Input: part model. Units: mm. Frame: model coordinates. Face numbers are marked on the shaded views. Give positions to 0.01 mm unless a question says otherwise; leave off trailing zeros. Loops run counter-clockwise (first coordinate to the right, second up) from the corner with the lowest first, then second, coordinate; pieces in that order, holes last. Notation, with made-up numbers: (-20.5, -29.5) - (-5.5, -29.5) arc R18 ccw to (-5.5, -17.5) - close; hole circle Ø8 at (21.5, 30). An arc over 180 degrees is marked (long way). Answer as a JSON object with one key per item and string values.
from build123d import *

# Parameters (mm, degrees)
SKETCH1_W           = 340.2
SKETCH1_H           = 155
BOSS_EXTRUDE1_DEPTH = 2
SKETCH2_R           = 2.5
CUT_EXTRUDE1_DEPTH  = 3
LPATTERN1_COUNT     = 4
LPATTERN1_PITCH     = 10
SKETCH3_W           = 59.862571915
SKETCH3_H           = 20.5
CUT_EXTRUDE2_DEPTH  = 3
LPATTERN2_COUNT     = 5
LPATTERN2_PITCH     = 10
SKETCH4_W           = 59.862571915
SKETCH4_H           = 9.012650354
CUT_EXTRUDE3_DEPTH  = 3
FILLET1_R           = 10
FILLET2_R           = 10
CUT_EXTRUDE4_DEPTH  = 3


with BuildPart() as part:
    # Sketch1 → Boss-Extrude1 (new body)
    with BuildSketch(Plane.XY):
        with Locations((440, -1022.5)):
            Rectangle(SKETCH1_W, SKETCH1_H)
    extrude(amount=BOSS_EXTRUDE1_DEPTH)

    # Sketch2 → Cut-Extrude1 (cut, through all)
    with BuildSketch(Plane.XY.offset(2)):
        with Locations((558.449514061, -1039.939996933)):
            Circle(SKETCH2_R)
        with Locations((349.784616085, -1041.525975933)):
            Circle(SKETCH2_R)
        with Locations((398.354490085, -962.715267)):
            Circle(SKETCH2_R)
        with Locations((549.405587829, -963.765953)):
            Circle(SKETCH2_R)
    cut_extrude1 = extrude(amount=-CUT_EXTRUDE1_DEPTH, mode=Mode.SUBTRACT)

    # LPattern1: Cut-Extrude1 ×4
    with Locations(*[(0, -i * LPATTERN1_PITCH, 0) for i in range(1, LPATTERN1_COUNT)]):
        add(cut_extrude1, mode=Mode.SUBTRACT)

    # Sketch3 → Cut-Extrude2 (cut, through all)
    with BuildSketch(Plane.XY.offset(2)):
        with Locations((440.285320332, -964.262650354)):
            Rectangle(SKETCH3_W, SKETCH3_H)
    cut_extrude2 = extrude(amount=-CUT_EXTRUDE2_DEPTH, mode=Mode.SUBTRACT)

    # LPattern2: Cut-Extrude2 ×5
    with Locations(*[(0, -i * LPATTERN2_PITCH, 0) for i in range(1, LPATTERN2_COUNT)]):
        add(cut_extrude2, mode=Mode.SUBTRACT)

    # Sketch4 → Cut-Extrude3 (cut, through all)
    with BuildSketch(Plane.XY.offset(2)):
        with Locations((440.285320332, -949.506325177)):
            Rectangle(SKETCH4_W, SKETCH4_H)
    extrude(amount=-CUT_EXTRUDE3_DEPTH, mode=Mode.SUBTRACT)

    # Fillet1
    fillet1_edges = [part.edges().sort_by_distance(p)[0] for p in [
        (470.216606289, -945, 1),
        (410.354034374, -945, 1),
        (410.354034374, -1014.512650354, 1),
        (470.216606289, -1014.512650354, 1),
    ]]
    fillet(fillet1_edges, radius=FILLET1_R)

    # Fillet2
    fillet2_edges = [part.edges().sort_by_distance(p)[0] for p in [
        (610.1, -1100, 1),
        (269.9, -1100, 1),
        (269.9, -945, 1),
        (610.1, -945, 1),
    ]]
    fillet(fillet2_edges, radius=FILLET2_R)

    # Sketch5 → Cut-Extrude4 (cut, through all)
    with BuildSketch(Plane.XY.offset(2)):
        with BuildLine():
            Line((523.449514061, -1075), (384.784616085, -1075))
            ThreePointArc((384.784616085, -1075), (381.249082179, -1073.535533906), (379.784616085, -1070))
            Line((379.784616085, -1070), (379.784616085, -1049.512650354))
            ThreePointArc((379.784616085, -1049.512650354), (381.249082179, -1045.977116448), (384.784616085, -1044.512650354))
            Line((384.784616085, -1044.512650354), (523.449514061, -1044.512650354))
            ThreePointArc((523.449514061, -1044.512650354), (526.985047967, -1045.977116448), (528.449514061, -1049.512650354))
            Line((528.449514061, -1049.512650354), (528.449514061, -1070))
            ThreePointArc((528.449514061, -1070), (526.985047967, -1073.535533906), (523.449514061, -1075))
        make_face()
        with BuildLine():
            Line((363.354490085, -1011.525975933), (304.9, -1011.525975933))
            ThreePointArc((304.9, -1011.525975933), (301.364466094, -1010.061509839), (299.9, -1006.525975933))
            Line((299.9, -1006.525975933), (299.9, -980))
            ThreePointArc((299.9, -980), (301.364466094, -976.464466094), (304.9, -975))
            Line((304.9, -975), (363.354490085, -975))
            ThreePointArc((363.354490085, -975), (366.890023991, -976.464466094), (368.354490085, -980))
            Line((368.354490085, -980), (368.354490085, -1006.525975933))
            ThreePointArc((368.354490085, -1006.525975933), (366.890023991, -1010.061509839), (363.354490085, -1011.525975933))
        make_face()
    extrude(amount=-CUT_EXTRUDE4_DEPTH, mode=Mode.SUBTRACT)


solid = part.part
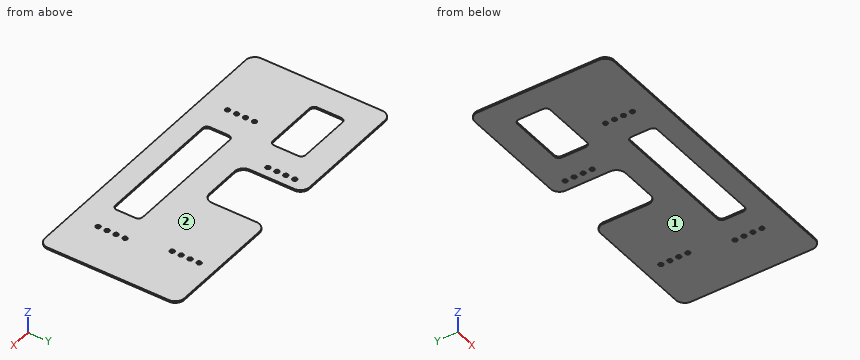
Item 1: Mould query, pull axis Z, two halves, no side actions, for the marked faces 1 and 2. Classes: released by +Z, released by -Z, zero draft, split by the parting line, or undercut.
Geometry check:
{"face 1": "released by -Z", "face 2": "released by +Z"}
Item 2: Material intervals for line 1 (X direction, y = -1002, z = 1.7); line 2 (Y direction, x = 421.5, z = 1); line 3 (X direction, y = -983, z = 0.2), sorted ascending. Write a range as [from, to].
Geometry check:
{"line 1": "x = [269.9, 299.9], [368.35, 410.35], [470.22, 610.1]", "line 2": "y = [-1100, -1075], [-1044.51, -1014.51]", "line 3": "x = [269.9, 299.9], [368.35, 395.87], [400.84, 410.35], [470.22, 547.03], [551.79, 610.1]"}
Item 3: Cut plane B-B (x = 317). Return loops of the section in (y, z), then the cut area to 3 significant figures.
Geometry check:
{"outline": "(-1100, 0) - (-1011.53, 0) - (-1011.53, 2) - (-1100, 2) - close; (-975, 0) - (-945, 0) - (-945, 2) - (-975, 2) - close", "area": "237 mm2"}
Item 4: Contact query for flat-ended pins moving along their axis: P1, Ø4, axis at x = 349.78, y = -1041.53, coming from the +Z side (3 decimals); P2, Ø0.6, axis at x = 444.5, z = 1, coming from the +Y side. Output: stop coordinate, or through.
Geometry check:
{"P1": "passes through", "P2": "stops at y = -1014.51"}
Item 5: Cut plane C-C (z = 1.2). Give the number of separate pieces and of enclosed holes in the cut face, then the cut area to 3 significant figures.
Geometry check:
{"separate pieces": "1", "enclosed holes": "18", "area": "41,200 mm2"}
Item 6: Cut plane A-A (x = 485.5). Return loops of the section in (y, z), then the cut area to 3 significant figures.
Geometry check:
{"outline": "(-1100, 0) - (-1075, 0) - (-1075, 2) - (-1100, 2) - close; (-1044.51, 0) - (-945, 0) - (-945, 2) - (-1044.51, 2) - close", "area": "249 mm2"}
